Could you check a few things on this model? Use its own coordinates, in mm. Face numbers are marked on the shaded views. A direction names the side the tool comes from. Coordinates: 2 decimals unless noted, no trailing zeros. Loops run counter-clockwise (first coordinate to the right, second up) from the corner with the lowest first, then second, coordinate; pieces in that order, holes last. Notation, with made-up numbers: (17.25, 10.5) -> (75.25, 10.5) arc R21 ccw to (75.25, 24.5) -> close; hole circle Ø2 at (43, -21). An arc over 180 degrees is marked (long way). One line per question, with ' | ' between items.
Autodesk Inventor part; units mm, degrees
ref_plane "YZ Plane" through (0, 0, 0) normal (1, 0, 0) x (0, 1, 0)
ref_plane "XZ Plane" through (0, 0, 0) normal (0, 1, 0) x (-1, 0, 0)
ref_plane "XY Plane" through (0, 0, 0) normal (0, 0, 1) x (1, 0, 0)
sketch "Sketch1" plane through (0, 0, 0) normal (0, 0, 1) x (1, 0, 0)
  line L0 (0, 0) -> (193.675, 0)
  line L1 (84.1375, 76.2) -> (109.5375, 76.2)
  line L2 (84.1375, 76.2) -> (29.0474, 0)
  line L3 (109.5375, 76.2) -> (164.6276, 0)
  line L4 (55.0901, 79.375) -> (1.1477, 4.7625)
  line L5 (138.5849, 79.375) -> (192.5273, 4.7625)
  line L6 (0, 0) -> (0, 3.175)
  line L7 (0, 3.175) -> (27.425, 3.175)
  line L8 (193.675, 0) -> (193.675, 3.175)
  line L9 (193.675, 3.175) -> (166.25, 3.175)
  line L10 (166.25, 3.175) -> (111.1599, 79.375)
  line L11 (111.1599, 79.375) -> (82.5151, 79.375)
  line L12 (82.5151, 79.375) -> (27.425, 3.175)
  line L13 (55.0901, 79.375) -> (82.5151, 79.375)
  line L14 (111.1599, 79.375) -> (138.5849, 79.375)
  line L15 (1.1477, 4.7625) -> (26.0399, 4.7625)
  line L16 (192.5273, 4.7625) -> (167.6351, 4.7625)
  arc A0 (26.0399, 3.175) -> (26.0399, 4.7625) centre (26.0399, 3.9688) ccw
  arc A1 (167.6351, 4.7625) -> (167.6351, 3.175) centre (167.6351, 3.9688) ccw
  dimension "d0" = 193.675
  dimension "d1" = 25.4
  dimension "d2" = 25.4
  dimension "d3" = 25.4
  dimension "d4" = 3.175
  dimension "d5" = 3.175
  dimension "d6" = 76.2
  dimension "d7" = 1.5875
  dimension "d8" = 1.5875
  dimension "d9" = 1.5875
extrude "Extrusion1" add sketch "Sketch1" along normal blind 25.4 contours L6 L7 L12 L11 L10 L9 L8 L0 L3 L1 L2
extrude "Extrusion2" add sketch "Sketch1" along normal blind 3.175 contours A0 L15 L4 L13 L12 L7 | L9 L10 L14 L5 L16 A1
fillet "Fillet1" radius 1.5875 4 edges at (166.25, 3.175, 14.2875) (27.425, 3.175, 14.2875) (84.1375, 76.2, 12.7) (109.5375, 76.2, 12.7)
fillet "Fillet2" radius 3.175 4 edges at (82.5151, 79.375, 14.2875) (111.1599, 79.375, 14.2875) (29.0474, 0, 12.7) (164.6276, 0, 12.7)
equation "\"d5\" = d4"
equation "\"d7\" = 0.5 * d4"
equation "\"d9\" = d8"
properties part number "bunny throw base 1"
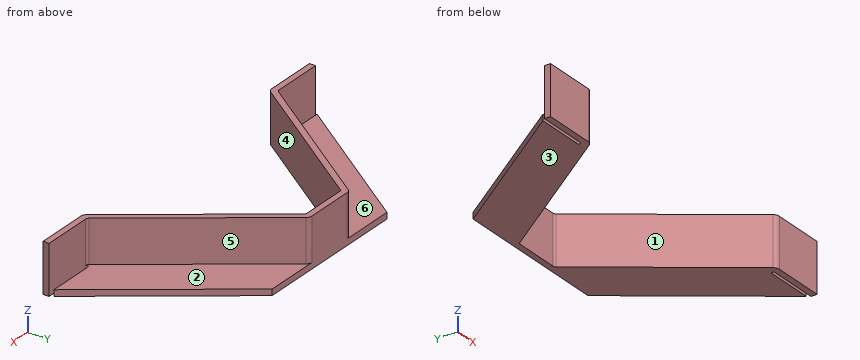
1) I'm going to push flat-ended pins straight in: pin 1 Ø7.5 at (x, z) = (17, 19) entering from +Y (3 decimals); pin 2 Ø6 at (y, z) = (41.5, 11) entering from +X; pin 3 Ø5 at (x, y) = (150, 60.5) entering from +Z (3 decimals). Where does each tip first touch, or does it pass through?
Data:
pin 1: y = 3.175 | pin 2: x = 140.71 | pin 3: z = 3.175
2) We'd pull the mould along X, two halves only. Please class the marked faces 4, 5 and 6: pulls with the +X half, pulls with the -X half, needs draft (parallel to the pull), parting line crosses it, or undercut.
Data:
face 4: undercut | face 5: pulls with the +X half | face 6: needs draft
3) I need wall thicknesses on line 1 along Y through (x, z) = (177, 18.5) (3 decimals); line 2 along X through (y, z) = (58, 8.75). Which ranges of each line are inside material? Lowest first, please. Write a range as from..to.
Data:
line 1: 0..3.175 | line 2: 67.06..70.98, 122.7..126.61
4) If we section it at B-B on x = 179.5: Please give me the cut outline in (y, z) (1 decimal).
Data:
outline: (0, 0) -> (3.2, 0) -> (3.2, 25.4) -> (0, 25.4) -> close; (4.8, 0) -> (22.8, 0) -> (22.8, 3.2) -> (4.8, 3.2) -> close
5) If we section it at A-A on y = 38.5: Please give me the cut outline in (x, z) (3 decimals).
Data:
outline: (25.539, 0) -> (56.882, 0) -> (56.882, 25.4) -> (52.964, 25.4) -> (52.964, 3.175) -> (25.539, 3.175) -> close; (136.793, 0) -> (168.136, 0) -> (168.136, 3.175) -> (140.711, 3.175) -> (140.711, 25.4) -> (136.793, 25.4) -> close
6) If we section it at D-D on x = 117: Please give me the cut outline in (y, z) (3 decimals).
Data:
outline: (65.878, 0) -> (79.375, 0) -> (79.375, 3.175) -> (71.297, 3.175) -> (71.297, 25.4) -> (65.878, 25.4) -> close
7) On a 3-axis mill with a long thin cutter (end or side, diameter ignored), from which of +Z, -Z, +X, -X, +Y, -Y can I reach the whole of each face in a straight line? I mean the marked faces 1, 2 and 3. Say none if no direction works.
Data:
face 1: +Z, -Z, -Y | face 2: +Z, +X, +Y | face 3: -Z, +X, -X, +Y, -Y
